Drawing for the job (mm, zero at the part's lowest x, y, z). A direction names the side the tool comes from. Give positions to 0.01 mm unless a question says otherwise; leave off trailing zeros. Write each loop counter-clockwise with the first axis right and the second up, starting at its lowest first coordinate (ties: lowest second). Pieces come first, ordered by that corner, then holes. Notation, with made-up numbers: M -38,45.25 L -13,45.25 A23 ccw -13,65.25 Z; hole C 65,66 d1. An arc over 180 degrees is marked long. Answer as a JSON object with one key per item and string values. Group by question number.
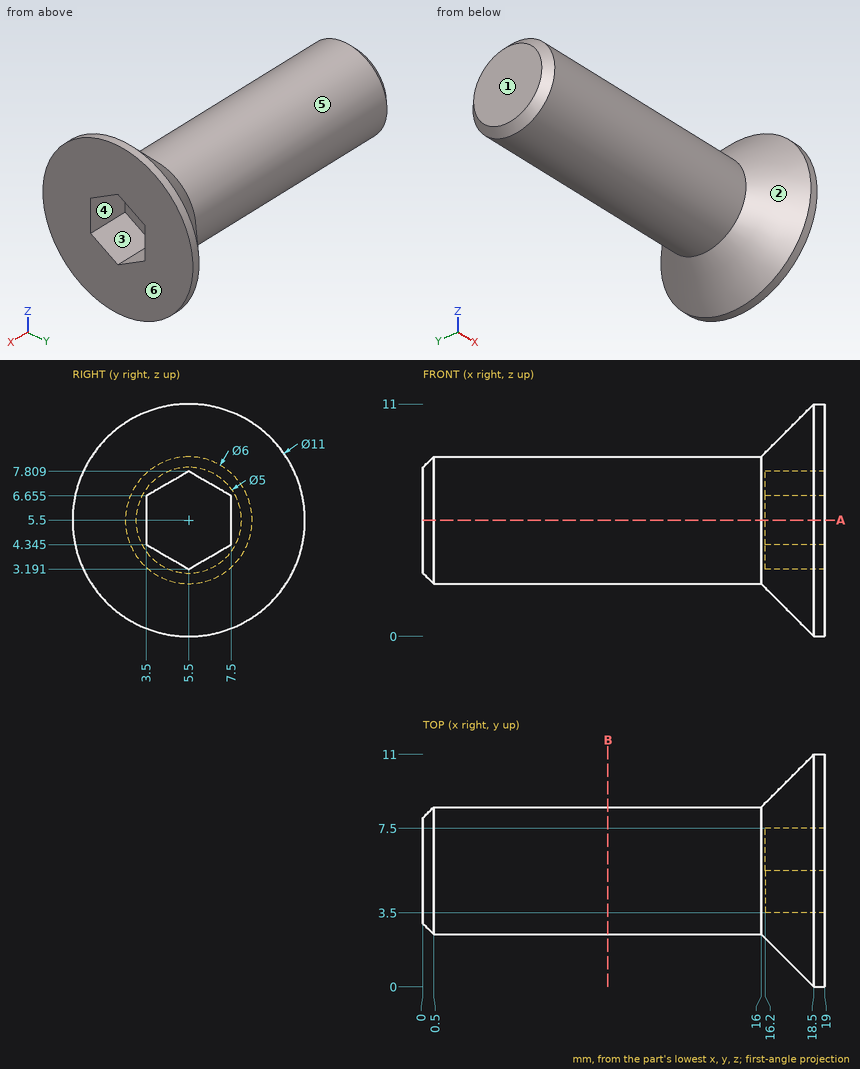
Q1. Slice it at A-A, the plane z = 5.5. Write the cut outline in (x, y).
Q2. 3-axis set-ups, long thin cutter, end or side, ignore diameter. For the marked faces 5 and 6: which of +Z, -Z, +X, -X, +Y, -Y reach the whole face in a straight line?
Q3. Drop flat-ended pins along their axis: P1, Ø2, axis at y = 6, z = 5, coming from the +X side; P2, Ø1, axis at y = 8.5, z = 5, coming from the -X side; P3, Ø0.7, axis at x = 17.5, z = 6, coming from the +Y side (1 decimal). Give the stop position or say it passes through.
Q4. Slice it at B-B, the plane x = 8.75. Write the cut outline in (y, z), then the cut area to 3 significant figures.
Q5. Wall check: L1, parallel to Y at x = 18, z = 6.5; L2, parallel to Z at x = 4.5, y = 5; L3, parallel to Y at x = 10.75, z = 8.25 (1 decimal). Give the ranges that are in metal, low to high.
Q6. Two-plate mould, pull along Y, no slides. Class the marked faces 1, 2, 3 and 4: +Y half, -Y half, draft (parallel to the pull), parting line (faces both ways), or undercut.
Solved:
{
 "1": {"outline": "M 0,3 L 0.5,2.5 L 16,2.5 L 18.5,0 L 19,0 L 19,3.5 L 16.2,3.5 L 16.2,7.5 L 19,7.5 L 19,11 L 18.5,11 L 16,8.5 L 0.5,8.5 L 0,8 Z"},
 "2": {"face 5": "-X", "face 6": "+Z, -Z, +X, +Y, -Y"},
 "3": {"P1": "stops at x = 16.2", "P2": "stops at x = 0.04", "P3": "stops at y = 10.3"},
 "4": {"outline": "C 5.5,5.5 d6", "area": "28.3 mm²"},
 "5": {"L1": "y = 0.6 to 3.5, 7.5 to 10.4", "L2": "z = 2.54 to 8.46", "L3": "y = 4.3 to 6.7"},
 "6": {"face 1": "draft", "face 2": "parting line", "face 3": "undercut", "face 4": "undercut"}
}
